Read the model definition and answer for the solid it produces. Units are mm, in the model's axes. Face numbers are marked on the shaded views. Round coordinates to 2 decimals unless told otherwise and drop trailing zeros. Write each loop counter-clockwise with the first axis right and the second up, starting at its lowest first coordinate (ties: lowest second). Pieces come first, ordered by that corner, then holes. Notation, with made-up numbers: (45, -25.5) - (95, -25.5) arc R10 cw to (95, -7.5) - close; hole circle Ø6 at (61.5, 8). An arc over 180 degrees is marked (long way). One line per item, written item: value. Start each with the question number.
(1) The mould has two halves that part along Y. Classify the marked faces 1 and 2: +Y half, -Y half, draft (parallel to the pull), parting line (faces both ways), or undercut.
(2) Find the intervals of material crossed by L1, parallel to Z at x = 2.5, y = 2.5; L2, parallel to Y at x = -2.75, z = 10; L3, parallel to Y at x = 1.35, z = 42.5, in increasing order.
(3) A cutting plane is placed at C-C, the plane y = 3. Determine the outline of the cut face in (x, z).
(4) A cutting plane is placed at B-B, the plane x = -8.5. State how many separate pieces and enclosed holes the cut face has, plus the area to 3 significant figures.
(5) A cutting plane is placed at D-D, the plane z = 31.5. Determine the outline of the cut face in (x, y), plus the area to 3 significant figures.
(6) Flat-ended cylindrical pins translate along their axes: pin 1 Ø2 at (y, z) = (-10, 132.5) entering from -X; pin 2 Ø4.5 at (x, z) = (-5, 113) entering from +Y; pin 3 Ø3 at (y, z) = (7.5, 132.5) entering from +X. Find the tip coordinate at first contact, or state that the pin passes through.
(7) A cutting plane is placed at A-A, the plane z = 75. Determine the outline of the cut face in (x, y).
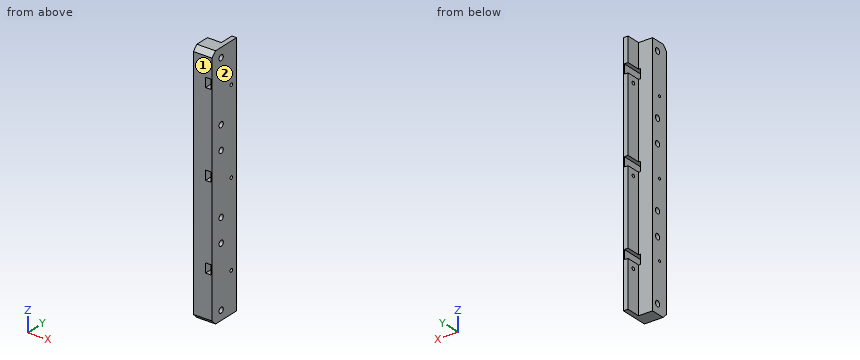
Autodesk Inventor part; units mm, degrees
ref_plane "YZ Plane" through (0, 0, 0) normal (1, 0, 0) x (0, 1, 0)
ref_plane "XZ Plane" through (0, 0, 0) normal (0, 1, 0) x (-1, 0, 0)
ref_plane "XY Plane" through (0, 0, 0) normal (0, 0, 1) x (1, 0, 0)
sketch "Sketch1" plane through (0, 0, 0) normal (0, 0, 1) x (1, 0, 0)
  line L0 (0, 0) -> (0, 15)
  line L1 (0, 15) -> (5, 15)
  line L2 (5, 15) -> (5, -20)
  line L3 (5, -20) -> (-15, -20)
  line L4 (-15, -20) -> (-15, 0)
  line L5 (-15, 0) -> (0, 0)
  dimension "d0" = 15
  dimension "d1" = 5
  dimension "d2" = 35
extrude "Extrusion1" add sketch "Sketch1" along normal blind 265
sketch "Sketch2" plane through (5, -20, 0) normal (1, 0, 0) x (0, 0, -1)
  line L0 (0, 0) -> (0, 35)
  line L1 (0, 35) -> (-265, 35)
  line L2 (-265, 0) -> (-265, 35)
  line L3 (0, 0) -> (-265, 0)
  point P0 (0, 20)
  point P1 (-222.5, 27.5)
  point P2 (-132.5, 27.5)
  point P3 (-42.5, 27.5)
  point P4 (-132.5, 35)
  dimension "d5" = 90
  dimension "d6" = 90
  dimension "d7" = 7.5
hole "Hole1" at (5, 7.5, 222.5) at (5, 7.5, 132.5) at (5, 7.5, 42.5) direction (-1, 0, 0) diameter 3.5 end through all
chamfer "Chamfer1" distance 5 angle 45 2 edges at (-5, -20, 265) (-5, -20, 0)
sketch "Sketch3" plane through (-15, 0, 0) normal (-1, 0, 0) x (0, 0, 1)
  line L0 (5, -20) -> (260, -20)
  line L1 (265, -15) -> (260, -20)
  line L2 (265, 0) -> (265, -15)
  line L3 (5, -20) -> (0, -15)
  line L4 (0, 0) -> (0, -15)
  line L5 (0, 0) -> (265, 0)
  point P0 (52.5, -10)
  point P1 (132.5, -10)
  point P2 (212.5, -10)
  point P3 (132.5, -20)
  dimension "d18" = 80
  dimension "d19" = 80
  dimension "d20" = 10
hole "Hole2" at (-15, -10, 52.5) at (-15, -10, 132.5) at (-15, -10, 212.5) direction (1, 0, 0) diameter 2.8 depth 15
sketch "Sketch4" plane through (5, 15, 265) normal (1, 0, 0) x (0, 0, -1)
  circle A0 centre (132.5, -7.5) radius 1.75
  circle A1 centre (42.5, -7.5) radius 1.75
  circle A2 centre (222.5, -7.5) radius 1.75
  line L0 (265, -30) -> (260, -35)
  line L1 (265, -30) -> (265, 0)
  line L2 (265, 0) -> (0, 0)
  line L3 (0, -30) -> (0, 0)
  line L4 (5, -35) -> (0, -30)
  line L5 (260, -35) -> (5, -35)
  point P0 (265, -15)
  point P1 (10, -22)
  point P2 (75, -22)
  point P3 (100, -22)
  point P4 (165, -22)
  point P5 (255, -22)
  point P6 (190, -22)
  dimension "d28" = 10
  dimension "d29" = 22
  dimension "d30" = 65
  dimension "d31" = 25
  dimension "d32" = 65
  dimension "d33" = 65
  dimension "d34" = 25
  dimension "d43" = 10
hole "Hole3" at (5, -7, 255) at (5, -7, 190) at (5, -7, 165) at (5, -7, 100) at (5, -7, 10) at (5, -7, 75) direction (-1, 0, 0) diameter 6 end through all
sketch "Sketch5" plane through (-15, -20, 5) normal (0, -1, 0) x (1, 0, 0)
  line L0 (20, 0) -> (0, 0)
  line L1 (20, 0) -> (20, 255)
  line L2 (0, 255) -> (20, 255)
  line L3 (0, 0) -> (0, 255)
  line L4 (15, 35.75) -> (15, 39.25)
  line L5 (20, 39.25) -> (20, 35.75)
  line L6 (15, 125.75) -> (15, 129.25)
  line L7 (20, 129.25) -> (20, 125.75)
  line L8 (15, 215.75) -> (15, 219.25)
  line L9 (20, 219.25) -> (20, 215.75)
  line L10 (19, 224.25) -> (13, 224.25)
  line L11 (13, 224.25) -> (13, 234.25)
  line L12 (13, 234.25) -> (19, 234.25)
  line L13 (19, 234.25) -> (19, 224.25)
  line L14 (19, 134.25) -> (13, 134.25)
  line L15 (13, 134.25) -> (13, 144.25)
  line L16 (13, 144.25) -> (19, 144.25)
  line L17 (19, 144.25) -> (19, 134.25)
  line L18 (19, 44.25) -> (13, 44.25)
  line L19 (13, 44.25) -> (13, 54.25)
  line L20 (13, 54.25) -> (19, 54.25)
  line L21 (19, 54.25) -> (19, 44.25)
  point P0 (15, -5)
  dimension "d44" = 1
  dimension "d45" = 5
  dimension "d46" = 5
  dimension "d47" = 5
  dimension "d48" = 10
  dimension "d49" = 6
extrude "Extrusion2" cut sketch "Sketch5" against normal through all contours L10 L11 L12 L13 | L14 L15 L16 L17 | L18 L19 L20 L21
equation "\"d46\" = d45"
equation "\"d47\" = d45"
properties part number "Toolhead Dock Assembly" material "ABS Plastic"
Here are the results:
1. face 1: -Y half
1. face 2: draft
2. L1: 0 to 49.25, 59.25 to 139.25, 149.25 to 229.25, 239.25 to 265
2. L2: -20 to -10, -4 to 0
2. L3: -20 to 5.75, 9.25 to 15
3. outline: (0, 0) - (5, 0) - (5, 265) - (0, 265) - (0, 239.25) - (4, 239.25) - (4, 229.25) - (0, 229.25) - (0, 149.25) - (4, 149.25) - (4, 139.25) - (0, 139.25) - (0, 59.25) - (4, 59.25) - (4, 49.25) - (0, 49.25) - close
4. separate pieces: 1
4. enclosed holes: 9
4. area: 5,090 mm²
5. outline: (-15, -20) - (5, -20) - (5, 15) - (0, 15) - (0, 0) - (-15, 0) - close
5. area: 475 mm²
6. pin 1: x = 0
6. pin 2: y = 0
6. pin 3: through
7. outline: (-15, -20) - (5, -20) - (5, -10) - (-15, -10) - close; (-15, -4) - (5, -4) - (5, 15) - (0, 15) - (0, 0) - (-15, 0) - close
